The model under review builds one solid part; all positions refer to its coordinate system, in mm. Face numbers are marked on the shaded views. Give positions to 0.01 mm unless a question says otherwise; leave off trailing zeros. Order: outer loops, then holes, each group sorted by start corner. A loop starts at its lowest first (then second) coordinate and runs counter-clockwise, first axis right, second up. Notation, with made-up numbers: M 33,-15 L 37,-15 A28 ccw 37,10 Z; hole C -12.75,32.25 d11. An arc over 180 degrees is marked long. One line per question, with ' | ' between items. Start each with the question number.
1. We need section A-A on x = 0. Write out the cut boundary in (y, z), then the cut area to 3 significant figures.
2. Wall thickness on L1, parallel to X at y = -2, z = 9.5; L2, parallel to Y at x = 15, z = 10.5; L3, parallel to Z at x = 1, y = -2.25: over which ranges is each line inside the solid? List them lowest first.
3. We need section C-C on y = 2. Write out the cut boundary in (x, z), then the cut area to 3 significant figures.
4. Insertion check: P1, Ø2, axis at y = 2, z = 11, coming from the +X side; P2, Ø5.5, axis at x = 0, z = -16.77, coming from the +Y side; P3, Ø1.5, axis at y = 2, z = -1.5, coming from the +X side. Each pin has a flat end and moves straight along its axis. Give the tip position at first contact, or say it passes through.
5. We need section B-B on y = -1. Write out the cut boundary in (x, z), then the cut area to 3 significant figures.
6. The part is to be moulded in two halves that separate along Z. For the marked faces 1, 2, 3 and 4, say which applies: +Z half, -Z half, draft (parallel to the pull), parting line (faces both ways), or undercut.
7. We need section D-D on z = 8. Count the separate pieces of the cut face and the enclosed holes in it, then the cut area to 3 significant figures.
```python
from build123d import *

# Parameters (mm, degrees)
SZKIC2_R                                             = 21.5
DODANIE_WYCI_GNI_CIE1_DEPTH                          = 3.3
DODANIE_WYCI_GNI_CIE1_OTHER_WAY_DEPTH                = 3
DODANIE_WYCI_GNI_CIE1_OTHER_WAY_TAPER                = 45
POG_BIENIE_WALCOWE_POD_M3_WKR_T_DO_CZ_CI_D           = 3.4
POG_BIENIE_WALCOWE_POD_M3_WKR_T_DO_CZ_CI_CBORE_D     = 7
POG_BIENIE_WALCOWE_POD_M3_WKR_T_DO_CZ_CI_CBORE_DEPTH = 2.4
SZYK_KO_OWY1_COUNT                                   = 3


with BuildPart() as part:
    # Szkic2 → Dodanie-wyciągnięcie1 (new body)
    with BuildSketch(Plane(origin=(0, 0, 0), x_dir=(1, 0, 0), z_dir=(0, 1, 0))):
        Circle(SZKIC2_R)
    extrude(amount=-DODANIE_WYCI_GNI_CIE1_DEPTH)

    # Szkic2 → Dodanie-wyciągnięcie1 other way (add)
    with BuildSketch(Plane(origin=(0, 0, 0), x_dir=(1, 0, 0), z_dir=(0, 1, 0))):
        Circle(SZKIC2_R)
    extrude(amount=DODANIE_WYCI_GNI_CIE1_OTHER_WAY_DEPTH, taper=DODANIE_WYCI_GNI_CIE1_OTHER_WAY_TAPER)

    # Pogłębienie walcowe pod M3 wkręt do części metalowych z łbem stożkowym ściętym2 (through all)
    with Locations(Plane(origin=(0, 3, 0), x_dir=(1, 0, 0), z_dir=(0, 1, 0))):
        with Locations((0, 16.772140565)):
            pog_bienie_walcowe_pod_m3_wkr_t_do_cz_ci = CounterBoreHole(POG_BIENIE_WALCOWE_POD_M3_WKR_T_DO_CZ_CI_D / 2, POG_BIENIE_WALCOWE_POD_M3_WKR_T_DO_CZ_CI_CBORE_D / 2, POG_BIENIE_WALCOWE_POD_M3_WKR_T_DO_CZ_CI_CBORE_DEPTH)

    # Szyk kołowy1: Pogłębienie walcowe pod M3 wkręt do części metalowych z łbem stożkowym ściętym2 ×3 about axis
    szyk_ko_owy1_axis = Axis((0, 0, 0), (0, 1, 0))
    for i in range(1, SZYK_KO_OWY1_COUNT):
        add(pog_bienie_walcowe_pod_m3_wkr_t_do_cz_ci.rotate(szyk_ko_owy1_axis, i * 360 / SZYK_KO_OWY1_COUNT), mode=Mode.SUBTRACT)


solid = part.part
```
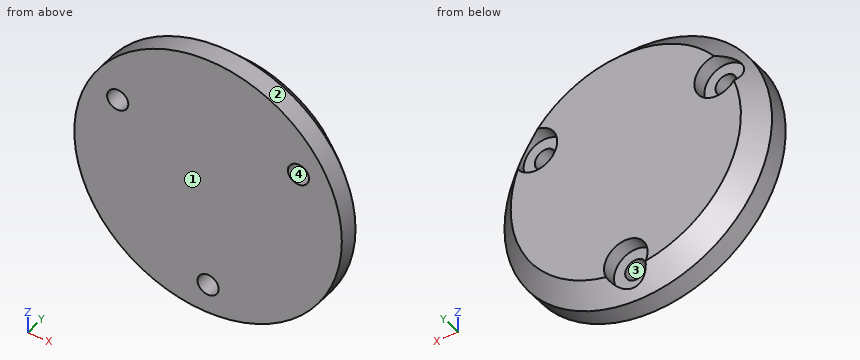
Entries:
1) outline: M -3.3,-21.5 L 0,-21.5 L 1.23,-20.27 L 0.6,-20.27 L 0.6,-18.47 L -3.3,-18.47 Z; M -3.3,-15.07 L 0.6,-15.07 L 0.6,-13.27 L 3,-13.27 L 3,18.5 L 0,21.5 L -3.3,21.5 Z | area: 233 mm^2
2) L1: x = -19.29 to -15.81, -13.24 to 13.24, 15.81 to 19.29 | L2: y = -3.3 to 0.6 | L3: z = -21.48 to -18.15, -15.4 to 21.48
3) outline: M -17.94,7.63 A19.5 ccw -2.36,-19.36 A3.5 cw long 2.36,-19.36 A19.5 ccw 17.94,7.63 A3.5 cw long 15.58,11.72 A19.5 ccw -15.58,11.72 A3.5 cw long Z | area: 1,090 mm^2
4) P1: stops at x = 17.45 | P2: stops at y = 0.6 | P3: stops at x = 20.2
5) outline: C 0,0 d43; hole C -14.53,8.39 d3.4; hole C 0,-16.77 d3.4; hole C 14.53,8.39 d3.4 | area: 1,420 mm^2
6) face 1: draft | face 2: parting line | face 3: undercut | face 4: undercut
7) separate pieces: 3 | enclosed holes: 0 | area: 184 mm^2
